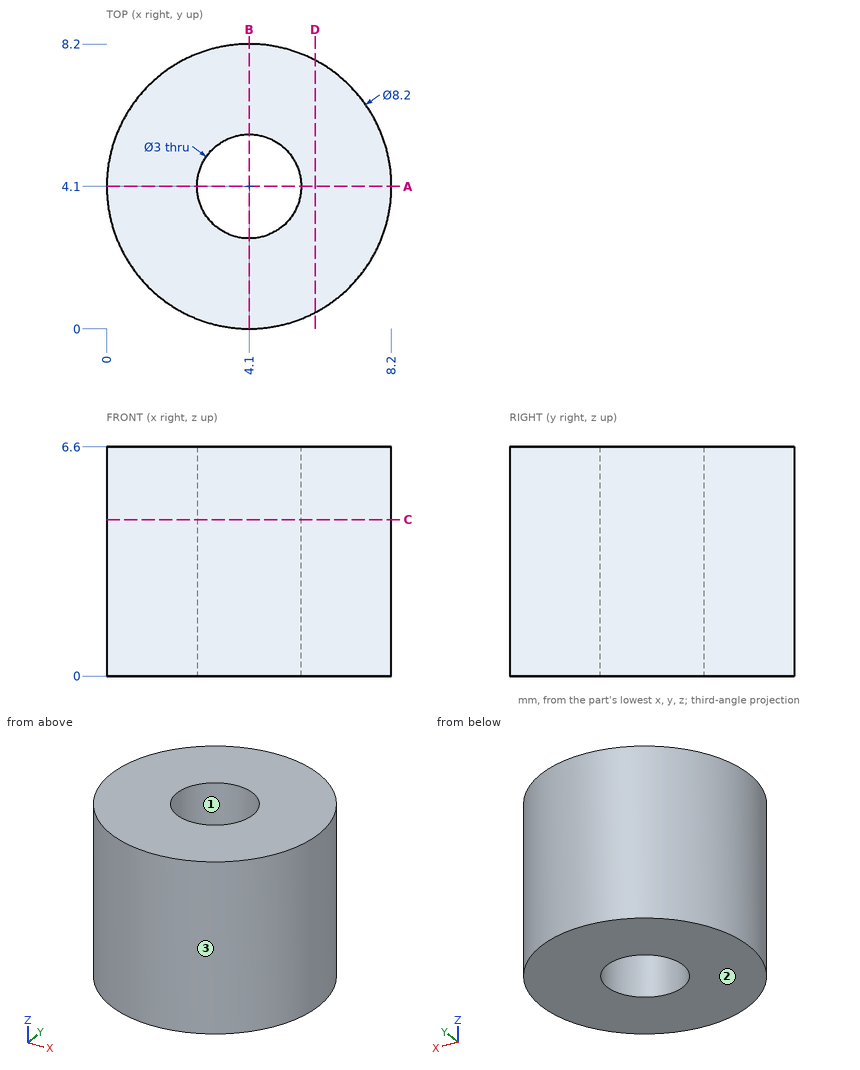
Geometry check sheet. Reference: drawing and pictorial views, mm from the part's lowest x, y, z. Coordinates: 2 decimals unless noted, no trailing zeros. Order: outer loops, then holes, each group sorted by start corner. A loop starts at its lowest first (then second) coordinate and runs counter-clockwise, first axis right, second up.
Item 1: Section check D-D (x = 6). Enter the section's corners in (y, z).
Item 2: Depth check by flat-ended pin: pin 1 (2 mm diameter, centred on x = 2, z = 5, fed in from -Y). Enter the tip coordinate at first touch or a pass-through.
Item 3: Scan lines: line 1 along Y through (x, z) = (4.1, 3); line 2 along Y through (x, z) = (3, 4). Record each from-to range of solid material in increasing order.
Item 4: Section check A-A (y = 4.1). Enter the section's corners in (x, z), plus the area to 3 significant figures.
Item 5: Mould release check, pull along X, two halves, no side actions. Record for the marked faces 1, 2 and 3: released by +X, released by -X, zero draft, split by the parting line, or undercut.
Item 6: Section check C-C (z = 4.5). Enter the section's corners in (x, y), plus the area to 3 significant figures.
Check sheet entries:
1. outline: (0.47, 0) - (7.73, 0) - (7.73, 6.6) - (0.47, 6.6) - close
2. pin 1: stops at y = 0.15
3. line 1: y = 0 to 2.6, 5.6 to 8.2
3. line 2: y = 0.15 to 3.08, 5.12 to 8.05
4. outline: (0, 0) - (2.6, 0) - (2.6, 6.6) - (0, 6.6) - close; (5.6, 0) - (8.2, 0) - (8.2, 6.6) - (5.6, 6.6) - close
4. area: 34.3 mm2
5. face 1: undercut
5. face 2: zero draft
5. face 3: split by the parting line
6. outline: circle Ø8.2 at (4.1, 4.1); hole circle Ø3 at (4.1, 4.1)
6. area: 45.7 mm2
